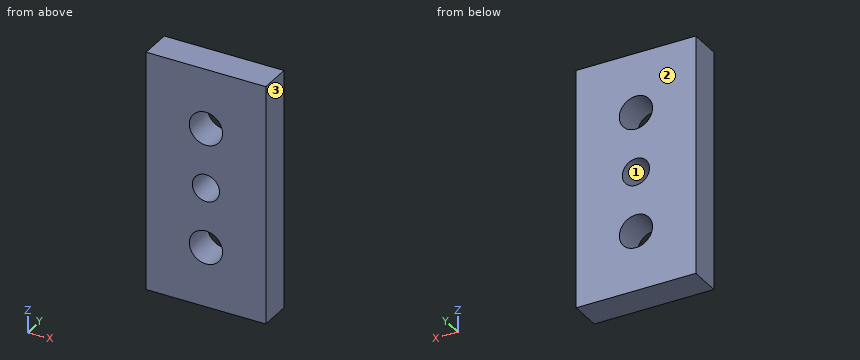
from build123d import *

# Parameters (mm, degrees)
SKETCH_1_W              = 45
SKETCH_1_H              = 90
SKETCH_1_R              = 6.25
EXTRUDE_1_DEPTH         = 12
HOLE_WIZARD_M12_1_D     = 10.2
HOLE_WIZARD_M12_1_DEPTH = 29.25
HOLE_WIZARD_M12_1_TIP   = 3.064389157


with BuildPart() as part:
    # 草图1 → 凸台-拉伸1 (new body)
    with BuildSketch(Plane(origin=(0, 0, 0), x_dir=(1, 0, 0), z_dir=(0, 1, 0))):
        with Locations((22.5, 45)):
            Rectangle(SKETCH_1_W, SKETCH_1_H)
        with Locations(Location((22.5, 67.5, 0), (0, 0, 270))):
            Circle(SKETCH_1_R, mode=Mode.SUBTRACT)
        with Locations(Location((22.5, 22.5, 0), (0, 0, 270))):
            Circle(SKETCH_1_R, mode=Mode.SUBTRACT)
    extrude(amount=EXTRUDE_1_DEPTH)

    # M12 螺纹孔1
    with Locations(Plane(origin=(22.5, 12, -45), x_dir=(0, 0, 1), z_dir=(0, 1, 0))):
        with Locations((0, 0)):
            Hole(HOLE_WIZARD_M12_1_D / 2, depth=HOLE_WIZARD_M12_1_DEPTH)
            with Locations((0, 0, -(HOLE_WIZARD_M12_1_DEPTH + HOLE_WIZARD_M12_1_TIP / 2))):  # 118° drill point
                Cone(0, HOLE_WIZARD_M12_1_D / 2, HOLE_WIZARD_M12_1_TIP, mode=Mode.SUBTRACT)


solid = part.part
Could you check a few things on this model? Use its own coordinates, in mm. Face numbers are marked on the shaded views. Coordinates: 2 decimals unless noted, no trailing zeros. Order: outer loops, then holes, each group sorted by start corner. A loop starts at its lowest first (then second) coordinate and runs counter-clockwise, first axis right, second up.
Q1. Will this pin go through, and if not, where does the flat tip stop? pin 1 (6 mm diameter, centred on x = 37.5, z = -33, fed in from -Y).
Q2. Suppose I cut it at B-B on z = -45. Please give me the cut outline in (x, y).
Q3. Suppose I cut it at D-D on z = -67.5. Please give me the cut outline in (x, y).
Q4. Thinking about a two-plate mould opening in X: for the marked faces 1, 2 and 3, which applies, released by +X, released by -X, zero draft, split by the parting line, or undercut?
Q5. Suppose I cut it at C-C on y = 5.5. Please give me the cut outline in (x, z).
Q6. Suppose I cut it at A-A on x = 22.5. Please give me the cut outline in (y, z).
Q7. Please list where these lines run through material, in increasing order: L1, parallel to X at y = 6.25, z = -67.5; L2, parallel to X at y = 7.25, z = -45; L3, parallel to Z at x = 22, y = 5.75.
Answer:
1. pin 1: stops at y = 0
2. outline: (0, 0) - (17.4, 0) - (17.4, 12) - (0, 12) - close; (27.6, 0) - (45, 0) - (45, 12) - (27.6, 12) - close
3. outline: (0, 0) - (16.25, 0) - (16.25, 12) - (0, 12) - close; (28.75, 0) - (45, 0) - (45, 12) - (28.75, 12) - close
4. face 1: undercut
4. face 2: zero draft
4. face 3: released by +X
5. outline: (0, -90) - (45, -90) - (45, 0) - (0, 0) - close; hole circle Ø12.5 at (22.5, -67.5); hole circle Ø12.5 at (22.5, -22.5); hole circle Ø10.2 at (22.5, -45)
6. outline: (0, -90) - (12, -90) - (12, -73.75) - (0, -73.75) - close; (0, -61.25) - (12, -61.25) - (12, -50.1) - (0, -50.1) - close; (0, -39.9) - (12, -39.9) - (12, -28.75) - (0, -28.75) - close; (0, -16.25) - (12, -16.25) - (12, 0) - (0, 0) - close
7. L1: x = 0 to 16.25, 28.75 to 45
7. L2: x = 0 to 17.4, 27.6 to 45
7. L3: z = -90 to -73.73, -61.27 to -50.08, -39.92 to -28.73, -16.27 to 0
